Geometry: final body of the model. Coordinates: model frame, mm. Coordinates: 2 decimals unless noted, no trailing zeros. Order: outer loops, then holes, each group sorted by start corner. A loop starts at its lowest first (then second) coordinate and runs counter-clockwise, first axis right, second up. Notation, with made-up numbers: (-31.75, 31.25) - (4.25, 31.25) arc R27 ccw to (4.25, 66.25) - close; hole circle Ø1 at (-5, 42). An arc over 180 degrees is marked (long way). Use a Markdown table: item, result. Add a question column.
```python
from build123d import *

# Parameters (mm, degrees)
SKETCH_1_W          = 32
SKETCH_1_H          = 38
EXTRUDE_1_DEPTH     = 2
SKETCH_2_R          = 10
CUT_EXTRUDE_1_DEPTH = 3
SKETCH_3_W          = 15
SKETCH_3_H          = 2
EXTRUDE_2_DEPTH     = 2
SKETCH_4_R          = 1.5
CUT_EXTRUDE_2_DEPTH = 3
SKETCH_5_R          = 1.6
CUT_EXTRUDE_3_DEPTH = 27.47640459


with BuildPart() as part:
    # 草图1 → 凸台-拉伸1 (new body)
    with BuildSketch(Plane.XY):
        Rectangle(SKETCH_1_W, SKETCH_1_H)
    extrude(amount=EXTRUDE_1_DEPTH)

    # 草图2 → 切除-拉伸1 (cut)
    with BuildSketch(Plane.XY.offset(2)):
        Circle(SKETCH_2_R)
    extrude(amount=-CUT_EXTRUDE_1_DEPTH, mode=Mode.SUBTRACT)

    # 草图3 → 凸台-拉伸2 (add)
    with BuildSketch(Plane.XY.offset(2)):
        with Locations((0, 20)):
            Rectangle(SKETCH_3_W, SKETCH_3_H)
        with Locations((0, -20)):
            Rectangle(SKETCH_3_W, SKETCH_3_H)
    extrude(amount=-EXTRUDE_2_DEPTH)

    # 草图4 → 切除-拉伸2 (cut)
    with BuildSketch(Plane.XY.offset(2)):
        with Locations((-9, 19)):
            Circle(SKETCH_4_R)
        with Locations((-9, -19)):
            Circle(SKETCH_4_R)
        with Locations((9, 19)):
            Circle(SKETCH_4_R)
        with Locations((9, -19)):
            Circle(SKETCH_4_R)
    extrude(amount=-CUT_EXTRUDE_2_DEPTH, mode=Mode.SUBTRACT)

    # 草图5 → 切除-拉伸3 (cut, through all)
    with BuildSketch(Plane.XY.offset(2)):
        with Locations((13.5, 16)):
            Circle(SKETCH_5_R)
        with Locations((13.5, -16)):
            Circle(SKETCH_5_R)
        with Locations(Location((-13.5, -16, 0), (0, 0, 180))):
            Circle(SKETCH_5_R)
        with Locations(Location((-13.5, 16, 0), (0, 0, 180))):
            Circle(SKETCH_5_R)
    extrude(amount=-CUT_EXTRUDE_3_DEPTH, mode=Mode.SUBTRACT)


solid = part.part
```
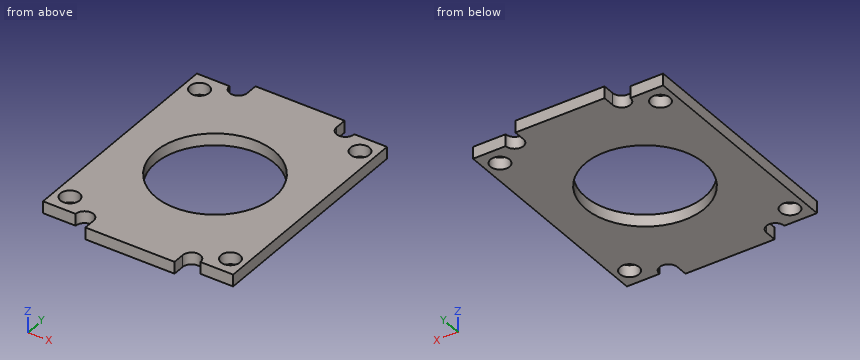
1) Section A-A (y = 8). Return loops of the section in (x, z), then the cut area to 3 significant figures.
2) Ray query, line 1 along Y through (x, z) = (-13.5, 0.8); line 2 along Y through (x, z) = (0, 1.3); line 3 along Y through (x, z) = (14, 1.4). Return the intervals inside material, ascending.
3) Section C-C (y = 16). Return loops of the section in (x, z).
4) Section D-D (z = 1.35). Return loops of the section in (x, y), then the cut area to 3 significant figures.
5) Section B-B (x = 0). Return loops of the section in (y, z).
6) Pin query (flat end, axial travel): pin 1 (0.6 mm diameter, centred on y = -19.5, z = 1.5, fed in from +X); pin 2 (0.6 mm diameter, centred on y = 20, z = 0.5, fed in from -X); pin 3 (1 mm diameter, centred on x = -12, z = 1.5, fed in from -Y). Return the tip coordinate at first contact, or that it passes through.
Values follow:
| question | item | result |
|---|---|---|
| 1 | outline | (-16, 0) - (-6, 0) - (-6, 2) - (-16, 2) - close; (6, 0) - (16, 0) - (16, 2) - (6, 2) - close |
| 1 | area | 40.0 mm² |
| 2 | line 1 | y = -19 to -17.6, -14.4 to 14.4, 17.6 to 19 |
| 2 | line 2 | y = -21 to -10, 10 to 21 |
| 2 | line 3 | y = -19 to -17.52, -14.48 to 14.48, 17.52 to 19 |
| 3 | outline | (-16, 0) - (-15.1, 0) - (-15.1, 2) - (-16, 2) - close; (-11.9, 0) - (11.9, 0) - (11.9, 2) - (-11.9, 2) - close; (15.1, 0) - (16, 0) - (16, 2) - (15.1, 2) - close |
| 4 | outline | (-16, -19) - (-10.5, -19) arc R1.5 cw to (-7.5, -19) - (-7.5, -21) - (7.5, -21) - (7.5, -19) arc R1.5 cw to (10.5, -19) - (16, -19) - (16, 19) - (10.5, 19) arc R1.5 cw to (7.5, 19) - (7.5, 21) - (-7.5, 21) - (-7.5, 19) arc R1.5 cw to (-10.5, 19) - (-16, 19) - close; hole circle Ø3.2 at (-13.5, -16); hole circle Ø3.2 at (-13.5, 16); hole circle Ø20 at (0, 0); hole circle Ø3.2 at (13.5, -16); hole circle Ø3.2 at (13.5, 16) |
| 4 | area | 916 mm² |
| 5 | outline | (-21, 0) - (-10, 0) - (-10, 2) - (-21, 2) - close; (10, 0) - (21, 0) - (21, 2) - (10, 2) - close |
| 6 | pin 1 | stops at x = 7.5 |
| 6 | pin 2 | stops at x = -7.5 |
| 6 | pin 3 | stops at y = -19 |
